Read the model definition and answer for the solid it produces. Units are mm, in the model's axes. A direction names the side the tool comes from. Coordinates: 2 decimals unless noted, no trailing zeros. Write each loop counter-clockwise with the first axis right and the second up, starting at its lowest first coordinate (ties: lowest second). Pieces come first, ordered by that corner, then holes. Notation, with made-up numbers: (66.25, 57) -> (90.25, 57) arc R8 ccw to (90.25, 72) -> close; hole circle Ø3 at (19, -16). An arc over 180 degrees is marked (long way). Answer as a JSON object with one key per item and string values. Group by question number.
(1) Straight lines are drawn through the part: L1, parallel to Y at x = 5.4, z = 0.85; L2, parallel to Y at x = 4, z = 0.8; L3, parallel to X at y = 7.5, z = 0.65. For each, find the intervals that lie inside material, in ascending order.
(2) Find section C-C (z = 1.15). Give the vertices of the cut face in (x, y), then the cut area to 3 significant figures.
(3) Which of the six approach directions +Z, -Z, +X, -X, +Y, -Y give full straight-line access (tool end or side, diameter ignored) to faces 1 (the face through (-1, 26.7, 1)), 2 (the face through (-1.95, 28, 1)), 3 (the face through (12, 26.7, 1))?
(4) Find section D-D (y = 10). Give the vertices of the cut face in (x, z).
(5) For a pull along X with two mould halves and no side action, classify faces 4 (the face through (12.18, 31.4, 1.04)), 5 (the face through (0, 15, 1)), 6 (the face through (7.02, 5.31, 1.04)), 7 (the face through (6.314, 26.433, 1.035)) as +X half, -X half, draft (parallel to the pull), parting line (faces both ways), or undercut.
(6) Find section A-A (x = 5.4). Give the vertices of the cut face in (y, z).
(7) Flat-ended cylindrical pins translate along their axes: P1, Ø1, axis at y = 20.5, z = 1.5, coming from the +X side; P2, Ø1, axis at x = 10.5, z = 1, coming from the -Y side. Find the tip coordinate at first contact, or state that the pin passes through.
(8) Find section B-B (y = 25). Give the vertices of the cut face in (x, z), then the cut area to 3 significant figures.
from build123d import *

# Parameters (mm, degrees)
SKETCH1_R           = 1.7
BOSS_EXTRUDE1_DEPTH = 2.1


with BuildPart() as part:
    # Sketch1 → Boss-Extrude1 (new body)
    with BuildSketch(Plane.XY):
        with BuildLine():
            ThreePointArc((0, 2), (0.585786438, 0.585786438), (2, 0))
            Line((2, 0), (8.8, 0))
            ThreePointArc((8.8, 0), (10.214213562, 0.585786438), (10.8, 2))
            Line((10.8, 2), (10.8, 26.7))
            Line((10.8, 26.7), (12.75, 26.7))
            Line((12.75, 26.7), (12.75, 30))
            ThreePointArc((12.75, 30), (12.164213562, 31.414213562), (10.75, 32))
            Line((10.75, 32), (0.05, 32))
            ThreePointArc((0.05, 32), (-1.364213562, 31.414213562), (-1.95, 30))
            Line((-1.95, 30), (-1.95, 26.7))
            Line((-1.95, 26.7), (0, 26.7))
            Line((0, 26.7), (0, 2))
        make_face()
        with Locations((5.4, 4.8)):
            Circle(SKETCH1_R, mode=Mode.SUBTRACT)
        with Locations((5.4, 25)):
            Circle(SKETCH1_R, mode=Mode.SUBTRACT)
    extrude(amount=BOSS_EXTRUDE1_DEPTH)


solid = part.part
Results below:
{
 "1": {"L1": "y = 0 to 3.1, 6.5 to 23.3, 26.7 to 32", "L2": "y = 0 to 3.84, 5.76 to 24.04, 25.96 to 32", "L3": "x = 0 to 10.8"},
 "2": {"outline": "(-1.95, 26.7) -> (0, 26.7) -> (0, 2) arc R2 ccw to (2, 0) -> (8.8, 0) arc R2 ccw to (10.8, 2) -> (10.8, 26.7) -> (12.75, 26.7) -> (12.75, 30) arc R2 ccw to (10.75, 32) -> (0.05, 32) arc R2 ccw to (-1.95, 30) -> close; hole circle Ø3.4 at (5.4, 4.8); hole circle Ø3.4 at (5.4, 25)", "area": "345 mm2"},
 "3": {"face 1": "+Z, -Z, -X, -Y", "face 2": "+Z, -Z, -X, +Y, -Y", "face 3": "+Z, -Z, +X, -Y"},
 "4": {"outline": "(0, 0) -> (10.8, 0) -> (10.8, 2.1) -> (0, 2.1) -> close"},
 "5": {"face 4": "+X half", "face 5": "-X half", "face 6": "undercut", "face 7": "undercut"},
 "6": {"outline": "(0, 0) -> (3.1, 0) -> (3.1, 2.1) -> (0, 2.1) -> close; (6.5, 0) -> (23.3, 0) -> (23.3, 2.1) -> (6.5, 2.1) -> close; (26.7, 0) -> (32, 0) -> (32, 2.1) -> (26.7, 2.1) -> close"},
 "7": {"P1": "stops at x = 10.8", "P2": "stops at y = 0.4"},
 "8": {"outline": "(0, 0) -> (3.7, 0) -> (3.7, 2.1) -> (0, 2.1) -> close; (7.1, 0) -> (10.8, 0) -> (10.8, 2.1) -> (7.1, 2.1) -> close", "area": "15.5 mm2"}
}
